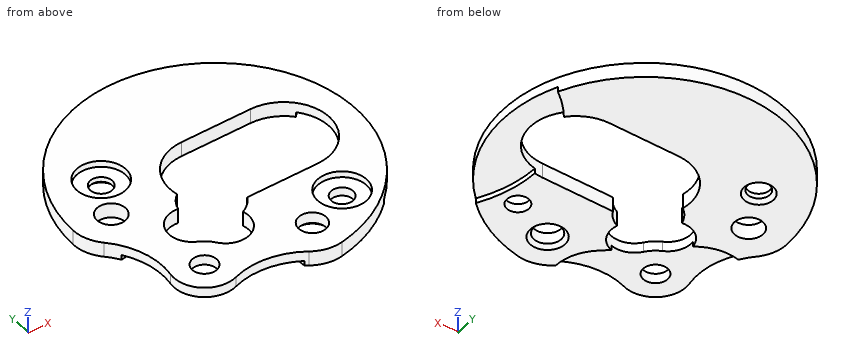
```python
from build123d import *
from OCP.BRepAlgoAPI import BRepAlgoAPI_Cut
from OCP.TopTools import TopTools_ListOfShape

# Parameters (mm, degrees)
BOSS_EXTRUDE1_DEPTH = 0.6
CUT_EXTRUDE1_DEPTH  = 0.2
SKETCH3_R           = 5.02
CUT_EXTRUDE2_DEPTH  = 0.2
HOLE1_D             = 1.162628638
HOLE2_D             = 1.115918006
HOLE3_D             = 1
HOLE3_DEPTH         = 0.6001
HOLE4_D             = 0.9
HOLE4_CBORE_D       = 2
HOLE4_CBORE_DEPTH   = 0.25
CHAMFER1_SIZE       = 0.15
FILLET1_R           = 1.55


with BuildPart() as part:
    # Sketch1 → Boss-Extrude1 (new body)
    with BuildSketch(Plane(origin=(0, 0, 0), x_dir=(-1, 0, 0), z_dir=(0, 0, -1))):
        with BuildLine():
            ThreePointArc((-10.73984142, -9.642233438), (-9.237924029, -8.831220946), (-7.536736276, -8.970710503))
            ThreePointArc((-7.536736276, -8.970710503), (-6.280146099, -8.76234417), (-5.858651118, -7.560355242))
            ThreePointArc((-5.858651118, -7.560355242), (-5.703315536, -5.860541144), (-4.645947853, -4.520589395))
            ThreePointArc((-4.645947853, -4.520589395), (-14.062387044, 0.497211479), (-10.73984142, -9.642233438))
        make_face()
        with BuildLine():
            Line((-10.362858107, -5.727073657), (-13.337303888, -5.648813517))
            ThreePointArc((-13.337303888, -5.648813517), (-15.131326546, -3.757835425), (-13.240348455, -1.963812767))
            Line((-13.240348455, -1.963812767), (-10.332680536, -2.040315926))
            ThreePointArc((-10.332680536, -2.040315926), (-8.949116824, -2.722465033), (-8.568642053, -4.217394763))
            ThreePointArc((-8.568642053, -4.217394763), (-8.294480547, -4.508437442), (-8.130929885, -4.873295708))
            ThreePointArc((-8.130929885, -4.873295708), (-7.112967422, -5.558507477), (-7.619937202, -6.675979798))
            ThreePointArc((-7.619937202, -6.675979798), (-7.888624675, -6.848520839), (-8.104829371, -7.083507857))
            ThreePointArc((-8.104829371, -7.083507857), (-9.292871814, -7.39061288), (-9.792686542, -6.269923994))
            ThreePointArc((-9.792686542, -6.269923994), (-10.123466132, -6.046492366), (-10.362858107, -5.727073657))
        make_face(mode=Mode.SUBTRACT)
    extrude(amount=-BOSS_EXTRUDE1_DEPTH)


with BuildPart() as cut_extrude1_tool:
    # Sketch2 → Cut-Extrude1 (new body)
    with BuildSketch(Plane(origin=(0, 0, 0), x_dir=(-1, 0, 0), z_dir=(0, 0, -1))):
        with BuildLine():
            Line((-9.182196127, -7.435630798), (-9.505531001, -7.707379249))
            ThreePointArc((-9.505531001, -7.707379249), (-10.019572014, -8.382539981), (-10.195186161, -9.212744683))
            ThreePointArc((-10.195186161, -9.212744683), (-8.894364476, -8.779749468), (-7.536736276, -8.97071434))
            ThreePointArc((-7.536736276, -8.97071434), (-6.280146099, -8.762348007), (-5.858651118, -7.560359079))
            ThreePointArc((-5.858651118, -7.560359079), (-5.86528742, -6.418236665), (-5.444571647, -5.356405283))
            ThreePointArc((-5.444571647, -5.356405283), (-6.302543189, -5.330829684), (-7.087113788, -5.678993801))
            ThreePointArc((-7.087113788, -5.678993801), (-7.189102384, -6.265354701), (-7.619937202, -6.675966608))
            ThreePointArc((-7.619937202, -6.675966608), (-7.888634149, -6.84851254), (-8.104845502, -7.083507857))
            ThreePointArc((-8.104845502, -7.083507857), (-8.585255131, -7.43783823), (-9.182196127, -7.435630798))
        make_face()
    extrude(amount=-CUT_EXTRUDE1_DEPTH)


with BuildPart() as part_1:
    add(part.part)

    # Cut-Extrude1: cut by cut_extrude1_tool, with a tolerance
    cut_extrude1_stock = TopTools_ListOfShape()
    cut_extrude1_stock.Append(part_1.part.wrapped)
    cut_extrude1_tools = TopTools_ListOfShape()
    cut_extrude1_tools.Append(cut_extrude1_tool.part.wrapped)
    cut_extrude1_cut = BRepAlgoAPI_Cut()
    cut_extrude1_cut.SetArguments(cut_extrude1_stock)
    cut_extrude1_cut.SetTools(cut_extrude1_tools)
    cut_extrude1_cut.SetFuzzyValue(0.00001)
    cut_extrude1_cut.Build()
    add(Compound.cast(cut_extrude1_cut.Shape()).solids(), mode=Mode.REPLACE)

    # Sketch3 → Cut-Extrude2 (cut)
    with BuildSketch(Plane(origin=(0, 0, 0), x_dir=(-1, 0, 0), z_dir=(0, 0, -1))):
        with Locations((-18.696793444, -5.59532139)):
            Circle(SKETCH3_R)
    extrude(amount=-CUT_EXTRUDE2_DEPTH, mode=Mode.SUBTRACT)

    # Sketch4 → Cut-Revolve1 (revolve, cut)
    with BuildSketch(Plane(origin=(0, -2.083255033, 0), x_dir=(1, 0, 0), z_dir=(0, 1, 0))):
        Polygon((7.58298739, 0), (6.98298739, 0), (6.98298739, -0.6), (7.98298739, -0.6), (7.98298739, -0.35), (7.43298739, -0.35), (7.43298739, -0.15), align=None)
    revolve(axis=Axis((6.98298739, -2.083255033, 0), (0, 0, 1)), mode=Mode.SUBTRACT)

    # Hole1 (through all)
    with Locations(Plane.XY.offset(0.6)):
        with Locations((6.16136425, -3.782231089)):
            Hole(HOLE1_D / 2)

    # Hole2 (through all)
    with Locations(Plane(origin=(0, 0, 0), x_dir=(-1, 0, 0), z_dir=(0, 0, -1))):
        with Locations((-11.320076522, -8.117897225)):
            Hole(HOLE2_D / 2)

    # Hole3
    with Locations(Plane.XY.offset(0.6)):
        with Locations((7.08439152, -7.80542761)):
            Hole(HOLE3_D / 2, depth=HOLE3_DEPTH)

    # Hole4 (through all)
    with Locations(Plane.XY.offset(0.6)):
        with Locations((13.162833859, -7.277138633)):
            CounterBoreHole(HOLE4_D / 2, HOLE4_CBORE_D / 2, HOLE4_CBORE_DEPTH)

    # Chamfer1
    chamfer1_edges = [part_1.edges().sort_by_distance(p)[0] for p in [
        (10.762117519, -8.117897225, 0),
    ]]
    chamfer(chamfer1_edges, length=CHAMFER1_SIZE)

    # Fillet1
    fillet1_edges = [part_1.edges().sort_by_distance(p)[0] for p in [
        (4.645947853, -4.520589395, 0.3),
        (10.73984142, -9.642233438, 0.3),
    ]]
    fillet(fillet1_edges, radius=FILLET1_R)


solid = part_1.part
```
Model file for the job. Use its own axes, mm. Coordinates: 2 decimals unless noted, no trailing zeros. Loops run counter-clockwise (first coordinate to the right, second up) from the corner with the lowest first, then second, coordinate; pieces in that order, holes last. Notation, with made-up numbers: M -17,47 L 3,47 A12 ccw 3,59 Z; hole C -1.75,-13 d3. An arc over 180 degrees is marked long. Use CSV: the item, a comma, the result in double quotes. Start each with the question number.
1. Probe probe 1 along Y at (x, z) = (7.5, 0.25); probe 2 along X at (y, z) = (-3.5, 0.55); probe 3 along Y at (x, z) = (13, 0.5) (3 decimals). List the from-to ranges inside material, lowest first. Write a range as [from, to].
2. Band-saw the part on A-A, the plane x = 15. List the corners of the cut face in (y, z), then the cut area to 3 significant figures.
3. Band-saw the part on B-B, the plane x = 13. List the corners of the cut face in (y, z) (3 decimals).
4. Band-saw the part on C-C, the plane x = 7.25. Give the number of separate pieces and of enclosed holes in the cut face, then the cut area to 3 significant figures.
5. Flat gauge pins, fed straight in: pin 1 (1 mm diameter, centred on x = 13, y = -7, fed in from +Z); pin 2 (6 mm diameter, centred on x = 9.5, y = -3.5, fed in from -Z); pin 3 (1.2 mm diameter, centred on x = 15.5, y = -6, fed in from -Z). Where does each tip first touch, or does it go through?
Entries:
1,probe 1,"y = [-8.98, -8.08], [-7.53, -6.61], [-5.03, 1.08]"
1,probe 2,"x = [4.63, 5.65], [6.67, 8.58], [15.11, 16.1]"
1,probe 3,"y = [-9.014, -8.264], [-6.29, -5.658], [-1.97, 1.205]"
2,outline,"M -7.3,0.2 L -4.49,0.2 L -4.49,0.6 L -7.3,0.6 Z; M -3.12,0.2 L -2.2,0.2 L -2.2,0 L -0.5,0 L -0.5,0.6 L -3.12,0.6 Z"
2,area,"2.51 mm2"
3,outline,"M -9.014,0 L -7.697,0 L -7.697,0.35 L -8.264,0.35 L -8.264,0.6 L -9.014,0.6 Z; M -6.858,0 L -5.658,0 L -5.658,0.6 L -6.29,0.6 L -6.29,0.35 L -6.858,0.35 Z; M -1.97,0 L 1.205,0 L 1.205,0.6 L -1.97,0.6 Z"
4,separate pieces,"4"
4,enclosed holes,"0"
4,area,"3.65 mm2"
5,pin 1,"stops at z = 0.35"
5,pin 2,"stops at z = 0"
5,pin 3,"stops at z = 0.2"
